Check sheet for the modelled part. Datum: model origin and axes. Units: mm. A direction names the side the tool comes from. Coordinates: 2 decimals unless noted, no trailing zeros. Loops run counter-clockwise (first coordinate to the right, second up) from the corner with the lowest first, then second, coordinate; pieces in that order, holes last. Notation, with made-up numbers: M 34.25,-37.75 L 51.25,-37.75 A6 ccw 51.25,-26.75 Z; hole C 60.25,59.25 d9. An arc over 180 degrees is marked long. Return JSON: item names as keys, results as strings.
from build123d import *

# Parameters (mm, degrees)
SKETCH1_W                 = 68.5
SKETCH1_H                 = 20
BOSS_EXTRUDE1_DEPTH       = 75
SKETCH5_W                 = 15
SKETCH5_H                 = 25
BOSS_EXTRUDE2_DEPTH       = 24
SKETCH6_R                 = 5.25
CUT_EXTRUDE4_DEPTH        = 46
SKETCH2_W                 = 44
SKETCH2_H                 = 44
CUT_EXTRUDE1_DEPTH        = 7
SKETCH3_R                 = 6.4135
SKETCH3_R_2               = 1.6
CUT_EXTRUDE2_DEPTH        = 14
SKETCH4_R                 = 12.5
CUT_EXTRUDE3_DEPTH        = 3
CHAMFER1_SIZE             = 1
FILLET1_R                 = 10
FILLET2_R                 = 5
SKETCH16_R                = 2.5796875
CUT_EXTRUDE6_DEPTH        = 20
SKETCH7_R                 = 2.5796875
CUT_EXTRUDE7_DEPTH        = 12.7
SKETCH7_3_R               = 5.7546875
SKETCH7_3_R_2             = 2.5796875
BOSS_EXTRUDE3_DEPTH       = 1.27
MIRROR3_COPY_1_SKETCH_R   = 2.5796875
MIRROR3_COPY_1_DEPTH      = 12.7
MIRROR3_COPY_2_SKETCH_R   = 5.7546875
MIRROR3_COPY_2_SKETCH_R_2 = 2.5796875
MIRROR3_COPY_2_DEPTH      = 1.27
CUT_EXTRUDE8_DEPTH        = 45


with BuildPart() as part:
    # Sketch1 → Boss-Extrude1 (new body)
    with BuildSketch(Plane(origin=(0, 0, 0), x_dir=(0, 0, -1), z_dir=(1, 0, 0))):
        with Locations((-34.25, 10)):
            Rectangle(SKETCH1_W, SKETCH1_H)
    boss_extrude1 = extrude(amount=BOSS_EXTRUDE1_DEPTH)

    # Mirror1: Boss-Extrude1 across plane
    add(boss_extrude1.mirror(Plane(origin=(75, 0, 68.5), x_dir=(1, 0, 0), z_dir=(0, 0, -1))))

    # Sketch5 → Boss-Extrude2 (add)
    with BuildSketch(Plane.XZ):
        with Locations((37.5, 68.5)):
            Rectangle(SKETCH5_W, SKETCH5_H)
    extrude(amount=BOSS_EXTRUDE2_DEPTH)

    # Sketch6 → Cut-Extrude4 (cut, through all)
    with BuildSketch(Plane.ZY.offset(-30)):
        with Locations((68.315835428, -12)):
            Circle(SKETCH6_R)
    extrude(amount=-CUT_EXTRUDE4_DEPTH, mode=Mode.SUBTRACT)

    # Sketch2 → Cut-Extrude1 (cut)
    with BuildSketch(Plane.XZ):
        with Locations((37.5, 109)):
            Rectangle(SKETCH2_W, SKETCH2_H)
    extrude(amount=-CUT_EXTRUDE1_DEPTH, mode=Mode.SUBTRACT)

    # Sketch3 → Cut-Extrude2 (cut, through all)
    with BuildSketch(Plane.XZ.offset(-7)):
        with Locations((37.5, 109)):
            Circle(SKETCH3_R)
        with Locations((22, 93.5)):
            Circle(SKETCH3_R_2)
        with Locations((22, 124.5)):
            Circle(SKETCH3_R_2)
        with Locations((53, 124.5)):
            Circle(SKETCH3_R_2)
        with Locations((53, 93.5)):
            Circle(SKETCH3_R_2)
    extrude(amount=-CUT_EXTRUDE2_DEPTH, mode=Mode.SUBTRACT)

    # Sketch4 → Cut-Extrude3 (cut)
    with BuildSketch(Plane.XZ.offset(-7)):
        with Locations((37.5, 109)):
            Circle(SKETCH4_R)
    extrude(amount=-CUT_EXTRUDE3_DEPTH, mode=Mode.SUBTRACT)

    # Chamfer1
    chamfer1_edges = [part.edges().sort_by_distance(p)[0] for p in [
        (51.4, 20, 93.5),
        (51.4, 20, 124.5),
        (20.4, 20, 124.5),
        (20.4, 20, 93.5),
    ]]
    chamfer(chamfer1_edges, length=CHAMFER1_SIZE)

    # Fillet1
    fillet1_edges = [part.edges().sort_by_distance(p)[0] for p in [
        (37.5, -24, 56),
        (37.5, -24, 81),
    ]]
    fillet(fillet1_edges, radius=FILLET1_R)

    # Fillet2
    fillet2_edges = [part.edges().sort_by_distance(p)[0] for p in [
        (30, 0, 68.5),
    ]]
    fillet(fillet2_edges, radius=FILLET2_R)

    # Sketch16 → Cut-Extrude6 (cut)
    with BuildSketch(Plane(origin=(0, 20, 0), x_dir=(1, 0, 0), z_dir=(0, 1, 0))):
        with Locations((37.5, -68.5)):
            Circle(SKETCH16_R)
    extrude(amount=-CUT_EXTRUDE6_DEPTH, mode=Mode.SUBTRACT)

    # Sketch7 → Cut-Extrude7 (cut)
    with BuildSketch(Plane(origin=(0, 0, 0), x_dir=(-1, 0, 0), z_dir=(0, 0, -1))):
        with Locations((-10, 7.874)):
            Circle(SKETCH7_R)
    cut_extrude7 = extrude(amount=-CUT_EXTRUDE7_DEPTH, mode=Mode.SUBTRACT)

    # Sketch7_3 → Boss-Extrude3 (add)
    with BuildSketch(Plane(origin=(0, 0, 0), x_dir=(-1, 0, 0), z_dir=(0, 0, -1))):
        with Locations((-10, 7.874)):
            Circle(SKETCH7_3_R)
        with Locations((-10, 7.874)):
            Circle(SKETCH7_3_R_2, mode=Mode.SUBTRACT)
    boss_extrude3 = extrude(amount=BOSS_EXTRUDE3_DEPTH)

    # Mirror2: Cut-Extrude7, Boss-Extrude3 across plane
    add(cut_extrude7.mirror(Plane.ZY.offset(-37.5)), mode=Mode.SUBTRACT)
    add(boss_extrude3.mirror(Plane.ZY.offset(-37.5)))

    # Mirror3: Boss-Extrude3, Cut-Extrude7 across plane
    add(boss_extrude3.mirror(Plane.XY.offset(68.5)))
    add(cut_extrude7.mirror(Plane.XY.offset(68.5)), mode=Mode.SUBTRACT)

    # Mirror3 copy 1 sketch → Mirror3 copy 1 (cut)
    with BuildSketch(Plane(origin=(75, 0, 137), x_dir=(1, 0, 0), z_dir=(0, 0, 1))):
        with Locations((-10, 7.874)):
            Circle(MIRROR3_COPY_1_SKETCH_R)
    extrude(amount=-MIRROR3_COPY_1_DEPTH, mode=Mode.SUBTRACT)

    # Mirror3 copy 2 sketch → Mirror3 copy 2 (add)
    with BuildSketch(Plane(origin=(75, 0, 137), x_dir=(1, 0, 0), z_dir=(0, 0, 1))):
        with Locations((-10, 7.874)):
            Circle(MIRROR3_COPY_2_SKETCH_R)
        with Locations((-10, 7.874)):
            Circle(MIRROR3_COPY_2_SKETCH_R_2, mode=Mode.SUBTRACT)
    extrude(amount=MIRROR3_COPY_2_DEPTH)

    # Sketch18 → Cut-Extrude8 (cut, through all)
    with BuildSketch(Plane(origin=(0, 20, 0), x_dir=(1, 0, 0), z_dir=(0, 1, 0))):
        Polygon((62.458777686, -88.720593409), (57.373918935, -83.400245236), (57.373918935, -39.549393127), (75, -20), (75, -121.613031971), (62.458777686, -108.491001941), align=None)
        Polygon((48.237394794, -32.421103895), (48.237394794, -52.62), (37.493383725, -52.62), (37.493383725, -7.62), (57.493383725, -7.62), (57.493383725, -22.155125557), align=None)
    cut_extrude8 = extrude(amount=-CUT_EXTRUDE8_DEPTH, mode=Mode.SUBTRACT)

    # Mirror4: Cut-Extrude8 across plane
    add(cut_extrude8.mirror(Plane.ZY.offset(-37.5)), mode=Mode.SUBTRACT)


solid = part.part
1) Draft check along Z on faces 6 (the face through (37.61, -20.99, 78.15)), 7 (the face through (62.459, 10, 99)), 8 (the face through (66.19, 5.585, 131.187)). Enter one of: +Z half, -Z half, draft (parallel to the pull), parting line (faces both ways), or undercut.
Answers:
{"face 6": "+Z half", "face 7": "undercut", "face 8": "draft"}
2) Section check B-B on z = 93.5. Record the cut outline in (x, y), then the cut area to 3 significant figures.
Answers:
{"outline": "M 12.54,0 L 15.5,0 L 15.5,7 L 20.4,7 L 20.4,19 L 19.4,20 L 12.54,20 Z; M 23.6,7 L 51.4,7 L 51.4,19 L 50.4,20 L 24.6,20 L 23.6,19 Z; M 54.6,7 L 59.5,7 L 59.5,0 L 62.46,0 L 62.46,20 L 55.6,20 L 54.6,19 Z", "area": "605 mm²"}
3) Go/stop test with flat-tipped pins: pin 1 Ø12 at (y, z) = (-1.5, 44) entering from -X; pin 2 Ø3.5 at (y, z) = (3, 101.5) entering from -X; pin 3 Ø4.5 at (x, y) = (65, 7.874) entering from +Z; pin 4 Ø2.5 at (x, z) = (22, 93.5) entering from -Y. Record where each tip stops, or that it passes through.
Answers:
{"pin 1": "x = 16.4", "pin 2": "x = 12.54", "pin 3": "z = 124.3", "pin 4": "through"}
4) Scan lines: line 1 along Z through (x, y) = (37.5, 14.25); line 2 along X through (y, z) = (12.5, 93.5); line 3 along X through (y, z) = (17.5, 47.5). Record each from-to range of solid material in increasing order. Write a range as [from, to].
Answers:
{"line 1": "[0, 7.62], [52.62, 65.92], [71.08, 102.59], [115.41, 137]", "line 2": "[12.54, 20.4], [23.6, 51.4], [54.6, 62.46]", "line 3": "[17.63, 26.76], [48.24, 57.37]"}
5) Set-up check for faces 1 (the face through (26.763, 10, 42)), 2 (the face through (35.873, 8.479, 121.394)), 3 (the face through (6.183, 10.14, 115.144)), 4 (the face through (45, -6, 68)), 5 (the face through (66.064, 10.14, 29.912)): record each of +Z, -Z, +X, -X, +Y, -Y from which the full face is reachable in a straight line by a thin tool's end or side.
Answers:
{"face 1": "+Y, -Y", "face 2": "-Y", "face 3": "-X, +Y, -Y", "face 4": "+Z, -Z, +X, -Y", "face 5": "+X, +Y, -Y"}
6) Section check D-D on x = 64. Record the cut outline in (y, z), then the cut area to 3 significant figures.
Answers:
{"outline": "M 0,0 L 2.21,0 L 2.21,-1.27 L 5.5,-1.27 L 5.5,12.7 L 10.25,12.7 L 10.25,-1.27 L 13.54,-1.27 L 13.54,0 L 20,0 L 20,32.2 L 0,32.2 Z; M 0,110.1 L 20,110.1 L 20,137 L 13.54,137 L 13.54,138.27 L 10.25,138.27 L 10.25,124.3 L 5.5,124.3 L 5.5,138.27 L 2.21,138.27 L 2.21,137 L 0,137 Z", "area": "1,080 mm²"}
7) Section check C-C on y = 16. Count the separate pieces of the cut face and the enclosed holes in it, then the cut area to 3 significant figures.
Answers:
{"separate pieces": "1", "enclosed holes": "7", "area": "6,050 mm²"}
8) Section check A-A on y = -12. Record the cut outline in (x, z).
Answers:
{"outline": "M 30,56 L 45,56 L 45,63.07 L 30,63.07 Z; M 30,73.57 L 45,73.57 L 45,81 L 30,81 Z"}
